Work out the finished part from the listing and answer in its coordinate system (mm). A direction names the side the tool comes from. Give positions to 0.01 mm unless a question says otherwise; leave off trailing zeros. Order: outer loops, then holes, each group sorted by start corner. A loop starts at its lowest first (then second) coordinate and runs counter-clockwise, first axis right, second up.
```python
from build123d import *

# Parameters (mm, degrees)
ESBO_O1_W                  = 30
ESBO_O1_H                  = 50
ESBO_O1_W_2                = 22
ESBO_O1_H_2                = 42
RESSALTO_EXTRUS_O1_DEPTH   = 20
ESBO_O3_R                  = 1.75
CORTE_EXTRUS_O2_DEPTH      = 44.874821937
ESBO_O4_W                  = 22
ESBO_O4_H                  = 9.5
ESBO_O4_R                  = 1.65
RESSALTO_EXTRUS_O2_DEPTH   = 4
CORTE_EXTRUS_O3_DEPTH      = 44.874821937
CORTE_EXTRUS_O3_DEPTH_BACK = 44.874821937


with BuildPart() as part:
    # Esboço1 → Ressalto-extrusão1 (new body)
    with BuildSketch(Plane(origin=(0, 0, 0), x_dir=(1, 0, 0), z_dir=(0, 1, 0))):
        Rectangle(ESBO_O1_W, ESBO_O1_H)
        Rectangle(ESBO_O1_W_2, ESBO_O1_H_2, mode=Mode.SUBTRACT)
    extrude(amount=RESSALTO_EXTRUS_O1_DEPTH)

    # Esboço3 → Corte-extrusão2 (cut, through all)
    with BuildSketch(Plane(origin=(15, 0, 0), x_dir=(0, 0, -1), z_dir=(1, 0, 0))):
        with Locations((-12, 15)):
            Circle(ESBO_O3_R)
        with Locations((12, 15)):
            Circle(ESBO_O3_R)
    extrude(amount=-CORTE_EXTRUS_O2_DEPTH, mode=Mode.SUBTRACT)

    # Esboço4 → Ressalto-extrusão2 (add)
    # profile 1 of 2: a face of its own
    with BuildSketch(Plane(origin=(0, 0, 0), x_dir=(1, 0, 0), z_dir=(0, 1, 0))):
        with Locations((0, 16.25)):
            Rectangle(ESBO_O4_W, ESBO_O4_H)
        with Locations(Location((-5, 15.5, 0), (0, 0, 270))):
            Circle(ESBO_O4_R, mode=Mode.SUBTRACT)
        with Locations(Location((5, 15.5, 0), (0, 0, 90))):
            Circle(ESBO_O4_R, mode=Mode.SUBTRACT)
    # profile 2 of 2: a face of its own
    with BuildSketch(Plane(origin=(0, 0, 0), x_dir=(1, 0, 0), z_dir=(0, 1, 0))):
        with Locations((0, -16.25)):
            Rectangle(ESBO_O4_W, ESBO_O4_H)
        with Locations(Location((5, -15.5, 0), (0, 0, 90))):
            Circle(ESBO_O4_R, mode=Mode.SUBTRACT)
        with Locations(Location((-5, -15.5, 0), (0, 0, 270))):
            Circle(ESBO_O4_R, mode=Mode.SUBTRACT)
    extrude(amount=RESSALTO_EXTRUS_O2_DEPTH)

    # Esboço5 → Corte-extrusão3 (cut, two sides: drawn at the far end of the back side and taken through both)
    with BuildSketch(Plane.ZY.offset(15).offset(-CORTE_EXTRUS_O3_DEPTH_BACK)):
        with BuildLine():
            Line((-16.736274298, 16.602406244), (-21, 4))
            Line((-21, 4), (-21, 0))
            Line((-21, 0), (-25, 0))
            Line((-25, 0), (-25, 4))
            Line((-25, 4), (-25, 20))
            Line((-25, 20), (-12, 20))
            ThreePointArc((-12, 20), (-14.914444096, 19.062759605), (-16.736274298, 16.602406244))
        make_face()
        with BuildLine():
            Line((25, 0), (25, 4))
            Line((25, 4), (25, 20))
            Line((25, 20), (12, 20))
            ThreePointArc((12, 20), (14.914444096, 19.062759605), (16.736274298, 16.602406244))
            Line((16.736274298, 16.602406244), (21, 4))
            Line((21, 4), (21, 0))
            Line((21, 0), (25, 0))
        make_face()
    extrude(amount=CORTE_EXTRUS_O3_DEPTH + CORTE_EXTRUS_O3_DEPTH_BACK, mode=Mode.SUBTRACT)


solid = part.part
```
1. Straight lines are drawn through the part: probe 1 along X at (y, z) = (2.9, -15.5); probe 2 along X at (y, z) = (3.25, 7.5); probe 3 along Z at (x, y) = (1.5, 2.5). For each, find the intervals that lie inside material, in ascending order.
Findings below:
probe 1: x = -15 to -6.65, -3.35 to 3.35, 6.65 to 15
probe 2: x = -15 to -11, 11 to 15
probe 3: z = -21 to -11.5, 11.5 to 21
2. The part is cut by section D-D (z = 2.5). Write down the section's boundary in (x, y), then the cut area to 3 significant figures.
Findings below:
outline: (-15, 0) - (-11, 0) - (-11, 20) - (-15, 20) - close; (11, 0) - (15, 0) - (15, 20) - (11, 20) - close
area: 160 mm2
3. The mould has two halves that part along Z. Classify faces 4 (the face through (0, 2, 11.5)), 5 (the face through (13, 19, -15)), 6 (the face through (13.03, 10.39, 18.84)), 7 (the face through (15, 10, 0)): pulls with the +Z half, pulls with the -Z half, needs draft (parallel to the pull), parting line crosses it, or undercut.
Findings below:
face 4: undercut
face 5: pulls with the -Z half
face 6: pulls with the +Z half
face 7: needs draft
4. Which of the six approach directions +Z, -Z, +X, -X, +Y, -Y give full straight-line access (tool end or side, diameter ignored) to faces 1 (the face through (0, 4, -16)), 2 (the face through (0, 2, -11.5)), 3 (the face through (13.028, 16.735, -11.772))?
Findings below:
face 1: +Z, -Z, +Y
face 2: +Y, -Y
face 3: +X, -X
5. The part is cut by section A-A (x = -5). Write down the section's boundary in (y, z), then the cut area to 3 significant figures.
Findings below:
outline: (0, -21) - (4, -21) - (4, -17.15) - (0, -17.15) - close; (0, -13.85) - (4, -13.85) - (4, -11.5) - (0, -11.5) - close; (0, 11.5) - (4, 11.5) - (4, 13.85) - (0, 13.85) - close; (0, 17.15) - (4, 17.15) - (4, 21) - (0, 21) - close
area: 49.6 mm2
6. Given P1, Ø12, axis at x = 11.5, y = 11, coming from the -Z side; P2, Ø2.5, axis at x = -5, z = 15.5, coming from the +Y side; P3, Ø7.5, axis at x = 2.5, z = 17.5, coming from the +Y side, each flat-ended and moving along its own axis, determine where each tip first touches the part or whether it passes through.
Findings below:
P1: stops at z = -20.66
P2: passes through
P3: stops at y = 4
7. The part is cut by section C-C (y = 7). Write down the section's boundary in (x, z).
Findings below:
outline: (-15, -19.99) - (-11, -19.99) - (-11, 19.99) - (-15, 19.99) - close; (11, -19.99) - (15, -19.99) - (15, 19.99) - (11, 19.99) - close
8. The part is cut by section B-B (z = -15.5). Write down the section's boundary in (x, y).
Findings below:
outline: (-15, 0) - (-6.65, 0) - (-6.65, 4) - (-11, 4) - (-11, 18.57) - (-15, 18.57) - close; (-3.35, 0) - (3.35, 0) - (3.35, 4) - (-3.35, 4) - close; (6.65, 0) - (15, 0) - (15, 18.57) - (11, 18.57) - (11, 4) - (6.65, 4) - close
